Geometry: final body of the model. Coordinates: model frame, mm. A direction names the side the tool comes from. Give positions to 0.01 mm unless a question says otherwise; leave off trailing zeros. Write each loop counter-clockwise with the first axis right and the second up, starting at its lowest first coordinate (ties: lowest second). Pieces come first, ordered by that corner, then holes. Notation, with made-up numbers: (13, -35) -> (70, -35) arc R25 cw to (70, -19) -> close; hole circle Ø4 at (-27.75, 46.25). An arc over 180 degrees is marked (long way). Answer as a JSON object with one key per item and string values.
Autodesk Inventor part; units mm, degrees
ref_plane "Work Plane1" through (0, 13.4219, 6.5) normal (0, 0, -1) x (-1, 0, 0)
ref_plane "YZ Plane" through (0, 0, 0) normal (1, 0, 0) x (0, 1, 0)
ref_plane "XZ Plane" through (0, 0, 0) normal (0, 1, 0) x (-1, 0, 0)
sketch "Sketch1" plane through (0, 0, 0) normal (0, 0, 1) x (1, 0, 0)
  line L0 (4, 0) -> (4, 3)
  line L1 (4, 3) -> (6.5, 6.1225)
  line L2 (6.5, 6.1225) -> (6.5, 12.1225)
  line L3 (6.5, 12.1225) -> (8, 12.1225)
  line L4 (8, 12.1225) -> (8, 3)
  line L5 (8, 3) -> (5, 3)
  line L6 (5, 3) -> (5, 0)
  line L7 (5, 0) -> (4, 0)
  line L8 (0, -2.6844) -> (0, 16.1063)
  point P0 (0, 0)
  dimension "d0" = 6.5
  dimension "d2" = 1.5
  dimension "d7" = 3
  dimension "d31" = 4
  dimension "d32" = 1
  dimension "d33" = 0
  dimension "d35" = 3
  dimension "d36" = 6
  dimension "d37" = 4
revolve "Revolution1" add sketch "Sketch1" angle 360 about axis through (0, -10, 0) along (0, 1, 0)
sketch "Sketch2" plane through (0, 0, 0) normal (1, 0, 0) x (0, 1, 0)
  line L0 (6.1225, 6.5) -> (12.1225, 6.5)
  point P0 (0, 0)
  point P1 (13.4219, 6.5)
ref_plane "Work Plane1" through (0, 13.4219, 6.5) normal (0, 0, -1) x (-1, 0, 0)
sketch "Sketch4" plane through (0, 0, 0) normal (1, 0, 0) x (0, 1, 0)
  line L0 (6.1225, 6.5) -> (6.1225, -6.5)
  line L1 (16.1063, 6.5) -> (-2.6844, 6.5)
  point P0 (0, 0)
  point P1 (7.6225, 6)
  dimension "d19" = 1.5
  dimension "d20" = 0.5
hole "Hole2" at (0, 7.6225, 6) direction (-1, 0, 0) diameter 1 end through all
pattern_circular "Circular Pattern1" count 6 over 360 about axis through (0, -10, 0) along (0, 1, 0) of "Hole2"
properties part number "bottom injector" material "Brass, Soft Yellow, Welded"
Q1. Cut plane B-B (y = 6.5). Return the cut outline in (x, z).
Values:
{"outline": "circle Ø16 at (0, 0); hole circle Ø13 at (0, 0)"}
Q2. Material intervals for L1, parallel to X at y = 9.75, z = 0; L2, parallel to X at y = 2.35, z = 0, sorted ascending. Write a range as from..to.
Values:
{"L1": "-8..-6.5, 6.5..8", "L2": "-5..-4, 4..5"}
Q3. Mould query, pull axis X, two halves, no side actions, for faces 1 (the flat face through (-0.1, 3, 5.2)), 2 (the cylindrical face through (3.69, 7.5, -7.1)), 3 (the cylindrical face through (-3.833, 7.601, -6.36)). Classes: pulls with the +X half, pulls with the -X half, needs draft (parallel to the pull), parting line crosses it, or undercut.
Values:
{"face 1": "needs draft", "face 2": "parting line crosses it", "face 3": "undercut"}
Q4. Set-up query: faces 4 (the cylindrical face through (-1.409, 9.164, 6.345)), 5 (the cylindrical face through (-3.6, 7.6, 6.5)), 6 (the cylindrical face through (-1.08, 1.48, -4.88)), 7 (the cylindrical face through (3.6, 7.6, -6.5)). Return all of +Z, -Z, +X, -X, +Y, -Y with unobstructed straight access to the full face (end or side cutting, diameter ignored); none if empty.
Values:
{"face 4": "+Y", "face 5": "-X", "face 6": "-Y", "face 7": "+X"}
Q5. Cut plane A-A (z = -6). State how many separate pieces and enclosed holes the cut face has, and give its area (3 significant figures).
Values:
{"separate pieces": "2", "enclosed holes": "1", "area": "60.8 mm²"}
Q6. First-contact query: P1, Ø1.5, axis at x = 1, y = 4, coming from the -Z side; P2, Ø2, axis at x = 6, y = 5.5, coming from the +Z side (3 decimals); P3, Ø3, axis at x = 3.5, z = 2.5, coming from the +Y side. Flat tips, straight axial feed; report the tip coordinate or a pass-through.
Values:
{"P1": "z = -8", "P2": "z = 6.245", "P3": "y = 5.25"}
